from build123d import *

# Parameters (mm, degrees)
BOSS_EXTRUDE1_DEPTH  = 2.5
BOSS_EXTRUDE6_DEPTH  = 24.5
CUT_EXTRUDE7_REACH   = 72.562
SKETCH3_R            = 2.5
BOSS_EXTRUDE11_START = -24.5
SKETCH12_R           = 1.4
BOSS_EXTRUDE11_DEPTH = 20
CUT_EXTRUDE11_REACH  = 120.55
SKETCH13_R           = 6.15
BOSS_EXTRUDE13_START = -4.5
SKETCH12_5_R         = 1.4
BOSS_EXTRUDE13_DEPTH = 2
CUT_EXTRUDE12_START  = -24.5
CUT_EXTRUDE12_DEPTH  = 24.5
BOSS_EXTRUDE14_START = -24.5
SKETCH12_6_R         = 1.4
BOSS_EXTRUDE14_DEPTH = 5


with BuildPart() as part:
    # Sketch1 → Boss-Extrude1 (new body)
    with BuildSketch(Plane(origin=(0, 0, 0), x_dir=(1, 0, 0), z_dir=(0, 1, 0))):
        with BuildLine():
            Line((-52, -35), (52, -35))
            ThreePointArc((52, -35), (54.121320344, -34.121320344), (55, -32))
            Line((55, -32), (55, 32))
            ThreePointArc((55, 32), (54.121320344, 34.121320344), (52, 35))
            Line((52, 35), (-52, 35))
            ThreePointArc((-52, 35), (-54.121320344, 34.121320344), (-55, 32))
            Line((-55, 32), (-55, -32))
            ThreePointArc((-55, -32), (-54.121320344, -34.121320344), (-52, -35))
        make_face()
    extrude(amount=-BOSS_EXTRUDE1_DEPTH)

    # Sketch7 → Boss-Extrude6 (add)
    with BuildSketch(Plane.XZ.offset(2.5)):
        with BuildLine():
            Line((-55, 32), (-55, -32))
            ThreePointArc((-55, -32), (-54.121320344, -34.121320344), (-52, -35))
            Line((-52, -35), (52, -35))
            ThreePointArc((52, -35), (54.121320344, -34.121320344), (55, -32))
            Line((55, -32), (55, 32))
            ThreePointArc((55, 32), (54.121320344, 34.121320344), (52, 35))
            Line((52, 35), (-52, 35))
            ThreePointArc((-52, 35), (-54.121320344, 34.121320344), (-55, 32))
        make_face()
        with BuildLine():
            Line((-53.5, 32), (-53.5, -32))
            ThreePointArc((-53.5, -32), (-53.060660172, -33.060660172), (-52, -33.5))
            Line((-52, -33.5), (52, -33.5))
            ThreePointArc((52, -33.5), (53.060660172, -33.060660172), (53.5, -32))
            Line((53.5, -32), (53.5, 32))
            ThreePointArc((53.5, 32), (53.060660172, 33.060660172), (52, 33.5))
            Line((52, 33.5), (-52, 33.5))
            ThreePointArc((-52, 33.5), (-53.060660172, 33.060660172), (-53.5, 32))
        make_face(mode=Mode.SUBTRACT)
    extrude(amount=BOSS_EXTRUDE6_DEPTH)

    # Sketch3 → Cut-Extrude7 (cut, up to next)
    with BuildSketch(Plane(origin=(0, 0, 0), x_dir=(1, 0, 0), z_dir=(0, 1, 0)), mode=Mode.PRIVATE) as cut_extrude7_sk1:
        with Locations(Location((-20.1, -27.5, 0), (0, 0, 270))):
            Circle(SKETCH3_R)
    cut_extrude7_tool1 = extrude(cut_extrude7_sk1.sketch, amount=-CUT_EXTRUDE7_REACH, mode=Mode.PRIVATE) & part.part
    # Sketch3 → Cut-Extrude7 (cut, up to next)
    with BuildSketch(Plane(origin=(0, 0, 0), x_dir=(1, 0, 0), z_dir=(0, 1, 0)), mode=Mode.PRIVATE) as cut_extrude7_sk2:
        with Locations(Location((-9.6, -27.5, 0), (0, 0, 270))):
            Circle(SKETCH3_R)
    cut_extrude7_tool2 = extrude(cut_extrude7_sk2.sketch, amount=-CUT_EXTRUDE7_REACH, mode=Mode.PRIVATE) & part.part
    # Sketch3 → Cut-Extrude7 (cut, up to next)
    with BuildSketch(Plane(origin=(0, 0, 0), x_dir=(1, 0, 0), z_dir=(0, 1, 0)), mode=Mode.PRIVATE) as cut_extrude7_sk3:
        with Locations(Location((0.5, -27.5, 0), (0, 0, 270))):
            Circle(SKETCH3_R)
    cut_extrude7_tool3 = extrude(cut_extrude7_sk3.sketch, amount=-CUT_EXTRUDE7_REACH, mode=Mode.PRIVATE) & part.part
    # Sketch3 → Cut-Extrude7 (cut, up to next)
    with BuildSketch(Plane(origin=(0, 0, 0), x_dir=(1, 0, 0), z_dir=(0, 1, 0)), mode=Mode.PRIVATE) as cut_extrude7_sk4:
        with Locations(Location((10.5, -27.5, 0), (0, 0, 270))):
            Circle(SKETCH3_R)
    cut_extrude7_tool4 = extrude(cut_extrude7_sk4.sketch, amount=-CUT_EXTRUDE7_REACH, mode=Mode.PRIVATE) & part.part
    add(cut_extrude7_tool1.solids().sort_by_distance((-20.1, 0, 27.5))[0], mode=Mode.SUBTRACT)
    add(cut_extrude7_tool2.solids().sort_by_distance((-9.6, 0, 27.5))[0], mode=Mode.SUBTRACT)
    add(cut_extrude7_tool3.solids().sort_by_distance((0.5, 0, 27.5))[0], mode=Mode.SUBTRACT)
    add(cut_extrude7_tool4.solids().sort_by_distance((10.5, 0, 27.5))[0], mode=Mode.SUBTRACT)

    # Sketch12 → Boss-Extrude11 (add)
    # profile 1 of 6: a face of its own
    with BuildSketch(Plane.XZ.offset(27).offset(BOSS_EXTRUDE11_START)):
        with BuildLine():
            Line((-39.5, 27.5), (-39.5, 33.5))
            Line((-39.5, 33.5), (-52, 33.5))
            ThreePointArc((-52, 33.5), (-53.060660172, 33.060660172), (-53.5, 32))
            Line((-53.5, 32), (-53.5, 22.5))
            Line((-53.5, 22.5), (-44.5, 22.5))
            ThreePointArc((-44.5, 22.5), (-40.964466094, 23.964466094), (-39.5, 27.5))
        make_face()
        with Locations(Location((-45.5, 27.5, 0), (0, 0, 270))):
            Circle(SKETCH12_R, mode=Mode.SUBTRACT)
    # profile 2 of 6: a face of its own
    with BuildSketch(Plane.XZ.offset(27).offset(BOSS_EXTRUDE11_START)):
        with BuildLine():
            Line((29.5, 33.5), (18.5, 33.5))
            Line((18.5, 33.5), (18.5, 27.5))
            ThreePointArc((18.5, 27.5), (19.964466094, 23.964466094), (23.5, 22.5))
            Line((23.5, 22.5), (24.5, 22.5))
            ThreePointArc((24.5, 22.5), (28.035533906, 23.964466094), (29.5, 27.5))
            Line((29.5, 27.5), (29.5, 33.5))
        make_face()
        with Locations(Location((24.5, 27.5, 0), (0, 0, 270))):
            Circle(SKETCH12_R, mode=Mode.SUBTRACT)
    # profile 3 of 6: a face of its own
    with BuildSketch(Plane.XZ.offset(27).offset(BOSS_EXTRUDE11_START)):
        with BuildLine():
            Line((18.5, -27.5), (18.5, -33.5))
            Line((18.5, -33.5), (29.5, -33.5))
            Line((29.5, -33.5), (29.5, -27.5))
            ThreePointArc((29.5, -27.5), (28.035533906, -23.964466094), (24.5, -22.5))
            Line((24.5, -22.5), (23.5, -22.5))
            ThreePointArc((23.5, -22.5), (19.964466094, -23.964466094), (18.5, -27.5))
        make_face()
        with Locations(Location((24.5, -27.5, 0), (0, 0, 270))):
            Circle(SKETCH12_R, mode=Mode.SUBTRACT)
    # profile 4 of 6: a face of its own
    with BuildSketch(Plane.XZ.offset(27).offset(BOSS_EXTRUDE11_START)):
        with BuildLine():
            Line((-44.5, -22.5), (-53.5, -22.5))
            Line((-53.5, -22.5), (-53.5, -32))
            ThreePointArc((-53.5, -32), (-53.060660172, -33.060660172), (-52, -33.5))
            Line((-52, -33.5), (-39.5, -33.5))
            Line((-39.5, -33.5), (-39.5, -27.5))
            ThreePointArc((-39.5, -27.5), (-40.964466094, -23.964466094), (-44.5, -22.5))
        make_face()
        with Locations(Location((-45.5, -27.5, 0), (0, 0, 270))):
            Circle(SKETCH12_R, mode=Mode.SUBTRACT)
    # profile 5 of 6: a face of its own
    with BuildSketch(Plane.XZ.offset(27).offset(BOSS_EXTRUDE11_START)):
        with BuildLine():
            Line((52, 33.5), (39.5, 33.5))
            Line((39.5, 33.5), (39.5, 27.5))
            ThreePointArc((39.5, 27.5), (40.964466094, 23.964466094), (44.5, 22.5))
            Line((44.5, 22.5), (53.5, 22.5))
            Line((53.5, 22.5), (53.5, 32))
            ThreePointArc((53.5, 32), (53.060660172, 33.060660172), (52, 33.5))
        make_face()
        with Locations(Location((45.5, 27.5, 0), (0, 0, 270))):
            Circle(SKETCH12_R, mode=Mode.SUBTRACT)
    # profile 6 of 6: a face of its own
    with BuildSketch(Plane.XZ.offset(27).offset(BOSS_EXTRUDE11_START)):
        with BuildLine():
            Line((53.5, -32), (53.5, -22.5))
            Line((53.5, -22.5), (44.5, -22.5))
            ThreePointArc((44.5, -22.5), (40.964466094, -23.964466094), (39.5, -27.5))
            Line((39.5, -27.5), (39.5, -33.5))
            Line((39.5, -33.5), (52, -33.5))
            ThreePointArc((52, -33.5), (53.060660172, -33.060660172), (53.5, -32))
        make_face()
        with Locations(Location((45.5, -27.5, 0), (0, 0, 270))):
            Circle(SKETCH12_R, mode=Mode.SUBTRACT)
    extrude(amount=BOSS_EXTRUDE11_DEPTH)

    # Sketch13 → Cut-Extrude11 (cut, up to next)
    with BuildSketch(Plane(origin=(55, 0, 0), x_dir=(0, 0, -1), z_dir=(1, 0, 0)), mode=Mode.PRIVATE) as cut_extrude11_sk1:
        with Locations((-12, -17)):
            Circle(SKETCH13_R)
    cut_extrude11_tool1 = extrude(cut_extrude11_sk1.sketch, amount=-CUT_EXTRUDE11_REACH, mode=Mode.PRIVATE) & part.part
    add(cut_extrude11_tool1.solids().sort_by_distance((55, -17, 12))[0], mode=Mode.SUBTRACT)

    # Sketch12<5> → Boss-Extrude13 (add)
    # profile 1 of 2: a face of its own
    with BuildSketch(Plane.XZ.offset(27).offset(BOSS_EXTRUDE13_START)):
        with BuildLine():
            Line((44.5, 22.5), (53.5, 22.5))
            Line((53.5, 22.5), (53.5, 32))
            ThreePointArc((53.5, 32), (53.060660172, 33.060660172), (52, 33.5))
            Line((52, 33.5), (39.5, 33.5))
            Line((39.5, 33.5), (39.5, 27.5))
            ThreePointArc((39.5, 27.5), (40.964466094, 23.964466094), (44.5, 22.5))
        make_face()
        with Locations(Location((45.5, 27.5, 0), (0, 0, 270))):
            Circle(SKETCH12_5_R, mode=Mode.SUBTRACT)
    # profile 2 of 2: a face of its own
    with BuildSketch(Plane.XZ.offset(27).offset(BOSS_EXTRUDE13_START)):
        with BuildLine():
            Line((39.5, -27.5), (39.5, -33.5))
            Line((39.5, -33.5), (52, -33.5))
            ThreePointArc((52, -33.5), (53.060660172, -33.060660172), (53.5, -32))
            Line((53.5, -32), (53.5, -22.5))
            Line((53.5, -22.5), (44.5, -22.5))
            ThreePointArc((44.5, -22.5), (40.964466094, -23.964466094), (39.5, -27.5))
        make_face()
        with Locations(Location((45.5, -27.5, 0), (0, 0, 270))):
            Circle(SKETCH12_5_R, mode=Mode.SUBTRACT)
    extrude(amount=BOSS_EXTRUDE13_DEPTH)

    # Sketch14 → Cut-Extrude12 (cut)
    with BuildSketch(Plane.XZ.offset(27).offset(CUT_EXTRUDE12_START)):
        with BuildLine():
            Line((-55, 32), (-55, -32))
            ThreePointArc((-55, -32), (-54.121320344, -34.121320344), (-52, -35))
            Line((-52, -35), (52, -35))
            ThreePointArc((52, -35), (54.121320344, -34.121320344), (55, -32))
            Line((55, -32), (55, 32))
            ThreePointArc((55, 32), (54.121320344, 34.121320344), (52, 35))
            Line((52, 35), (-52, 35))
            ThreePointArc((-52, 35), (-54.121320344, 34.121320344), (-55, 32))
        make_face()
    extrude(amount=CUT_EXTRUDE12_DEPTH, mode=Mode.SUBTRACT)

    # Sketch12<6> → Boss-Extrude14 (add)
    with BuildSketch(Plane.XZ.offset(27).offset(BOSS_EXTRUDE14_START)):
        with Locations(Location((-45.5, 27.5, 0), (0, 0, 270))):
            Circle(SKETCH12_6_R)
        with Locations(Location((-45.5, -27.5, 0), (0, 0, 270))):
            Circle(SKETCH12_6_R)
        with Locations(Location((24.5, -27.5, 0), (0, 0, 270))):
            Circle(SKETCH12_6_R)
        with Locations(Location((45.5, -27.5, 0), (0, 0, 270))):
            Circle(SKETCH12_6_R)
        with Locations(Location((45.5, 27.5, 0), (0, 0, 270))):
            Circle(SKETCH12_6_R)
        with Locations(Location((24.5, 27.5, 0), (0, 0, 270))):
            Circle(SKETCH12_6_R)
    extrude(amount=BOSS_EXTRUDE14_DEPTH)


solid = part.part
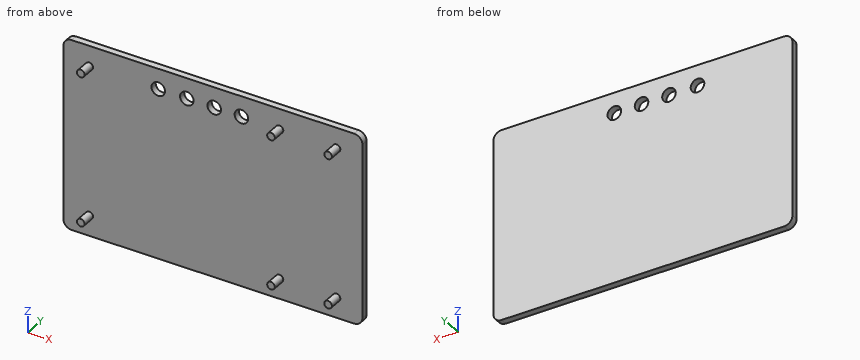
For this review, take the finished solid that the model builds, in its own axes (mm). Coordinates: 2 decimals unless noted, no trailing zeros. Order: outer loops, then holes, each group sorted by start corner. A loop starts at its lowest first (then second) coordinate and runs counter-clockwise, first axis right, second up. Notation, with made-up numbers: (-19, 2.25) -> (9, 2.25) arc R27 ccw to (9, 26.25) -> close; hole circle Ø4 at (83.25, 17.25). An arc over 180 degrees is marked (long way). Return JSON: item names as keys, results as strings.
1. We need section D-D on x = 24.5. Write out the cut boundary in (y, z), and give its area (3 significant figures).
Answer block:
{"outline": "(-7.5, -28.9) -> (-2.5, -28.9) -> (-2.5, -35) -> (0, -35) -> (0, 35) -> (-2.5, 35) -> (-2.5, 28.9) -> (-7.5, 28.9) -> (-7.5, 26.1) -> (-2.5, 26.1) -> (-2.5, -26.1) -> (-7.5, -26.1) -> close", "area": "203 mm²"}
2. For line 1 (X direction, y = -1.55, z = 27.5); line 2 (Y direction, x = -27, z = -9); line 3 (X direction, y = -1.75, z = 29.5), list the stretches that pass through material, from the lowest coordinate up. Write a range as from..to.
Answer block:
{"line 1": "-55..-22.6, -17.6..-12.1, -7.1..-2, 3..8, 13..55", "line 2": "-2.5..0", "line 3": "-55..-21.6, -18.6..-11.1, -8.1..-1, 2..9, 12..55"}
3. We need section A-A on x = 10.5. Write out the cut boundary in (y, z).
Answer block:
{"outline": "(-2.5, -35) -> (0, -35) -> (0, 25) -> (-2.5, 25) -> close; (-2.5, 30) -> (0, 30) -> (0, 35) -> (-2.5, 35) -> close"}
4. We need section C-C on y = -4. Write out the cut boundary in (x, z), and give its area (3 significant figures).
Answer block:
{"outline": "circle Ø2.8 at (-45.5, -27.5); circle Ø2.8 at (-45.5, 27.5); circle Ø2.8 at (24.5, -27.5); circle Ø2.8 at (24.5, 27.5); circle Ø2.8 at (45.5, -27.5); circle Ø2.8 at (45.5, 27.5)", "area": "36.9 mm²"}
5. For pin 1 Ø1 at (y, z) = (-5, 26) entering from +X; pin 2 Ø21 at (x, z) = (20, 8) entering from -Y, all flat-tipped, find the tip position at first contact; note any pin that passes through.
Answer block:
{"pin 1": "x = 46.48", "pin 2": "y = -2.5"}
6. We need section B-B on z = -27.5. Write out the cut boundary in (x, y).
Answer block:
{"outline": "(-55, -2.5) -> (-46.9, -2.5) -> (-46.9, -7.5) -> (-44.1, -7.5) -> (-44.1, -2.5) -> (23.1, -2.5) -> (23.1, -7.5) -> (25.9, -7.5) -> (25.9, -2.5) -> (44.1, -2.5) -> (44.1, -7.5) -> (46.9, -7.5) -> (46.9, -2.5) -> (55, -2.5) -> (55, 0) -> (-55, 0) -> close"}
